Could you check a few things on this model? Use its own coordinates, in mm. Face numbers are marked on the shaded views. A direction names the side the tool comes from. Round coordinates to 2 decimals unless told otherwise and drop trailing zeros. Order: outer loops, then holes, each group sorted by start corner. A loop starts at its lowest first (then second) coordinate and runs counter-clockwise, first axis right, second up. Notation, with made-up numbers: (57.25, 16.5) -> (88.25, 16.5) arc R26 ccw to (88.25, 36.5) -> close; hole circle Ø6 at (86.5, 34.25). An arc over 180 degrees is marked (long way). One line per question, with ' | ' between items.
```python
from build123d import *

# Parameters (mm, degrees)
F1_DEPTH  = 38.1
F3_DEPTH  = 273.05
F4_W      = 25.4
F4_H      = 38.1
F4_W_2    = 50.8
F5_DEPTH  = 12.7
F7_DEPTH  = 38.1
F8_R      = 2.54
F10_DEPTH = 11.049
F11_DEPTH = 11.049
F12_DEPTH = 63.5
F13_SIZE  = 19.05


with BuildPart() as f1:
    # F0 (on Top) → F1 (new body)
    with BuildSketch(Plane.XY):
        Polygon((-63.5, -152.4), (63.5, -152.4), (63.5, 88.9), (63.5, 101.6), (63.5, 114.3), (63.5, 152.4), (-63.5, 152.4), (-63.5, 114.3), (-63.5, 101.6), (-63.5, 88.9), align=None)
    extrude(amount=F1_DEPTH)

    # F2 (on face) → F3 (cut)
    with BuildSketch(Plane.XZ.offset(152.4)):
        Polygon((-12.7, 0), (0, 0), (12.7, 0), (12.7, 16.51), (31.75, 16.51), (31.75, 29.21), (12.7, 29.21), (12.7, 38.1), (-12.7, 38.1), (-12.7, 29.21), (-31.75, 29.21), (-31.75, 16.51), (-12.7, 16.51), align=None)
    extrude(amount=-F3_DEPTH, mode=Mode.SUBTRACT)

    # F4 (on face) → F5 (join)
    with BuildSketch(Plane.XY.offset(38.1)):
        with Locations((0, -133.35)):
            Rectangle(F4_W, F4_H)
        with Locations((-38.1, -133.35)):
            Rectangle(F4_W_2, F4_H)
        with Locations((38.1, -133.35)):
            Rectangle(F4_W_2, F4_H)
    extrude(amount=F5_DEPTH)

    # F6 (on face) → F7 (join)
    with BuildSketch(Plane.XZ.offset(152.4)):
        with BuildLine():
            Line((-47.625, 50.8), (0, 50.8))
            Line((0, 50.8), (47.625, 50.8))
            Line((47.625, 50.8), (21.0934256055, 90.3501730104))
            ThreePointArc((21.0934256055, 90.3501730104), (0, 101.6), (-21.0934256055, 90.3501730104))
            Line((-21.0934256055, 90.3501730104), (-47.625, 50.8))
        make_face()
        with BuildLine():
            ThreePointArc((12.7, 76.2), (8.9802561211, 67.2197438789), (0, 63.5))
            ThreePointArc((0, 63.5), (-8.9802561211, 85.1802561211), (12.7, 76.2))
        make_face(mode=Mode.SUBTRACT)
    extrude(amount=-F7_DEPTH)

    # F8
    f8_edges = [f1.edges().sort_by_distance(p)[0] for p in [
        (-55.5625, -152.4, 50.8),
        (55.5625, -152.4, 50.8),
        (34.359213, -152.4, 70.575087),
        (63.5, -133.35, 50.8),
        (-55.5625, -114.3, 50.8),
        (55.5625, -114.3, 50.8),
        (34.359213, -114.3, 70.575087),
        (0, -152.4, 101.6),
        (0, -114.3, 101.6),
        (-34.359213, -152.4, 70.575087),
        (-34.359213, -114.3, 70.575087),
        (-63.5, -133.35, 50.8),
    ]]
    fillet(f8_edges, radius=F8_R)

    # F0 (on Top) → F10 (join)
    with BuildSketch(Plane.XY):
        with BuildLine():
            Line((-88.9, 88.9), (-63.5, 88.9))
            Line((-63.5, 88.9), (-63.5, 101.6))
            Line((-63.5, 101.6), (-69.977, 101.6))
            ThreePointArc((-69.977, 101.6), (-70.9441334085, 99.2651334085), (-73.279, 98.298))
            Line((-73.279, 98.298), (-76.6367705722, 98.298))
            ThreePointArc((-76.6367705722, 98.298), (-81.1748915865, 91.5196875048), (-88.9, 88.9))
        make_face()
        with BuildLine():
            Line((-69.977, 101.6), (-63.5, 101.6))
            Line((-63.5, 101.6), (-63.5, 114.3))
            Line((-63.5, 114.3), (-88.9, 114.3))
            ThreePointArc((-88.9, 114.3), (-81.1748915865, 111.6803124952), (-76.6367705722, 104.902))
            Line((-76.6367705722, 104.902), (-73.279, 104.902))
            ThreePointArc((-73.279, 104.902), (-70.9441334085, 103.9348665915), (-69.977, 101.6))
        make_face()
        with BuildLine():
            Line((-88.9, 98.298), (-88.9, 88.9))
            ThreePointArc((-88.9, 88.9), (-81.1748915865, 91.5196875048), (-76.6367705722, 98.298))
            Line((-76.6367705722, 98.298), (-88.9, 98.298))
        make_face()
        with BuildLine():
            ThreePointArc((-101.6, 101.6), (-97.8802561211, 92.6197438789), (-88.9, 88.9))
            Line((-88.9, 88.9), (-88.9, 98.298))
            ThreePointArc((-88.9, 98.298), (-91.2348665915, 99.2651334085), (-92.202, 101.6))
            Line((-92.202, 101.6), (-101.6, 101.6))
        make_face()
        with BuildLine():
            ThreePointArc((-88.9, 114.3), (-97.8802561211, 110.5802561211), (-101.6, 101.6))
            Line((-101.6, 101.6), (-92.202, 101.6))
            ThreePointArc((-92.202, 101.6), (-91.2348665915, 103.9348665915), (-88.9, 104.902))
            Line((-88.9, 104.902), (-88.9, 114.3))
        make_face()
        with BuildLine():
            ThreePointArc((-76.6367705722, 104.902), (-81.1748915865, 111.6803124952), (-88.9, 114.3))
            Line((-88.9, 114.3), (-88.9, 104.902))
            Line((-88.9, 104.902), (-76.6367705722, 104.902))
        make_face()
    extrude(amount=F10_DEPTH)

    # F0 (on Top) → F11 (join)
    with BuildSketch(Plane.XY):
        with BuildLine():
            Line((63.5, 101.6), (63.5, 88.9))
            Line((63.5, 88.9), (88.9, 88.9))
            ThreePointArc((88.9, 88.9), (81.1748915865, 91.5196875048), (76.6367705722, 98.298))
            Line((76.6367705722, 98.298), (73.279, 98.298))
            ThreePointArc((73.279, 98.298), (70.9441334085, 99.2651334085), (69.977, 101.6))
            Line((69.977, 101.6), (63.5, 101.6))
        make_face()
        with BuildLine():
            ThreePointArc((76.6367705722, 98.298), (81.1748915865, 91.5196875048), (88.9, 88.9))
            Line((88.9, 88.9), (88.9, 98.298))
            Line((88.9, 98.298), (76.6367705722, 98.298))
        make_face()
        with BuildLine():
            Line((92.202, 101.6), (101.6, 101.6))
            ThreePointArc((101.6, 101.6), (97.8802561211, 110.5802561211), (88.9, 114.3))
            Line((88.9, 114.3), (88.9, 104.902))
            ThreePointArc((88.9, 104.902), (91.2348665915, 103.9348665915), (92.202, 101.6))
        make_face()
        with BuildLine():
            Line((88.9, 98.298), (88.9, 88.9))
            ThreePointArc((88.9, 88.9), (97.8802561211, 92.6197438789), (101.6, 101.6))
            Line((101.6, 101.6), (92.202, 101.6))
            ThreePointArc((92.202, 101.6), (91.2348665915, 99.2651334085), (88.9, 98.298))
        make_face()
        with BuildLine():
            Line((88.9, 104.902), (88.9, 114.3))
            ThreePointArc((88.9, 114.3), (81.1748915865, 111.6803124952), (76.6367705722, 104.902))
            Line((76.6367705722, 104.902), (88.9, 104.902))
        make_face()
        with BuildLine():
            Line((63.5, 114.3), (63.5, 101.6))
            Line((63.5, 101.6), (69.977, 101.6))
            ThreePointArc((69.977, 101.6), (70.9441334085, 103.9348665915), (73.279, 104.902))
            Line((73.279, 104.902), (76.6367705722, 104.902))
            ThreePointArc((76.6367705722, 104.902), (81.1748915865, 111.6803124952), (88.9, 114.3))
            Line((88.9, 114.3), (63.5, 114.3))
        make_face()
    extrude(amount=F11_DEPTH)

    # F9 (on face) → F12 (join)
    with BuildSketch(Plane.XY.offset(38.1)):
        Polygon((-63.5, 120.65), (-12.7, 120.65), (12.7, 120.65), (63.5, 120.65), (63.5, 152.4), (-63.5, 152.4), align=None)
    extrude(amount=F12_DEPTH)

    # F13
    f13_edges = [f1.edges().sort_by_distance(p)[0] for p in [
        (0, 152.4, 101.6),
    ]]
    chamfer(f13_edges, length=F13_SIZE)


solid = f1.part
```
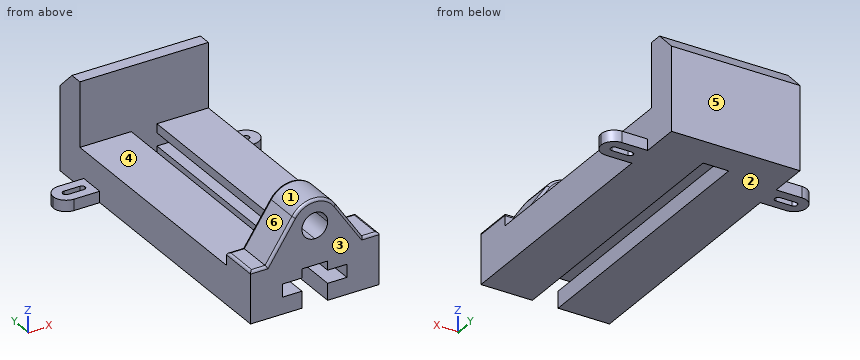
1. I'm going to push flat-ended pins straight in: pin 1 (5.5 mm diameter, centred on x = -77.5, z = 4, fed in from -Y); pin 2 (5.5 mm diameter, centred on x = -80.5, z = 7.5, fed in from +Y); pin 3 (8 mm diameter, centred on x = -38, y = 55.5, fed in from +Z); pin 4 (10 mm diameter, centred on x = 69.5, z = 36.5, fed in from +Y). Where does each tip first touch, or does it pass through?
From the geometry:
pin 1: stops at y = 88.9 | pin 2: stops at y = 114.3 | pin 3: stops at z = 38.1 | pin 4: passes through
2. If we mould it in two halves opening along Z, with no side actions, what happens to the marked faces 1, 2 and 3? For each: pulls with the +Z half, pulls with the -Z half, needs draft (parallel to the pull), parting line crosses it, or undercut.
From the geometry:
face 1: pulls with the +Z half | face 2: pulls with the -Z half | face 3: needs draft
3. I want a section at B-B on x = -51.5. List the corners of the cut face in (y, z) for me, and give its area (3 significant figures).
From the geometry:
outline: (-152.4, 0) -> (152.4, 0) -> (152.4, 82.55) -> (133.35, 101.6) -> (120.65, 101.6) -> (120.65, 38.1) -> (-114.3, 38.1) -> (-114.3, 48.26) arc R2.54 ccw to (-116.84, 50.8) -> (-149.86, 50.8) arc R2.54 ccw to (-152.4, 48.26) -> close | area: 13,900 mm²
4. On a 3-axis mill with a long thin cutter (end or side, diameter ignored), from which of +Z, -Z, +X, -X, +Y, -Y can I reach the whole of each face in a straight line? I mean the marked faces 4, 5 and 6. Say none if no direction works.
From the geometry:
face 4: +Z, +X, -X | face 5: +Z, -Z, +X, -X, +Y | face 6: +Z, -X, -Y
5. I want a section at A-A on y = 61. List the corners of the cut face in (x, z) for me, and give its area (3 significant figures).
From the geometry:
outline: (-63.5, 0) -> (-12.7, 0) -> (-12.7, 16.51) -> (-31.75, 16.51) -> (-31.75, 29.21) -> (-12.7, 29.21) -> (-12.7, 38.1) -> (-63.5, 38.1) -> close; (12.7, 0) -> (63.5, 0) -> (63.5, 38.1) -> (12.7, 38.1) -> (12.7, 29.21) -> (31.75, 29.21) -> (31.75, 16.51) -> (12.7, 16.51) -> close | area: 3,390 mm²
6. I want a section at C-C on z = 24. List the corners of the cut face in (x, y) for me, and give its area (3 significant figures).
From the geometry:
outline: (-63.5, -152.4) -> (-31.75, -152.4) -> (-31.75, 120.65) -> (31.75, 120.65) -> (31.75, -152.4) -> (63.5, -152.4) -> (63.5, 152.4) -> (-63.5, 152.4) -> close | area: 21,400 mm²
7. I need wall thicknesses on probe 1 along Z at (x, y) = (27, -106); probe 2 along X at (y, z) = (15.5, 8); probe 3 along Y at (x, z) = (22, 51). Which ranges of each line are inside material? Lowest first, please.
From the geometry:
probe 1: z = 0 to 16.51, 29.21 to 38.1 | probe 2: x = -63.5 to -12.7, 12.7 to 63.5 | probe 3: y = -152.4 to -114.3, 120.65 to 152.4
8. I want a section at D-D on x = -8. Count the separate pieces of the cut face and the enclosed holes in it, and give its area (3 significant figures).
From the geometry:
separate pieces: 3 | enclosed holes: 0 | area: 4,660 mm²
